The figure shows three views and two pictorial views of one solid part (mm, origin at its lowest corner). Answer the questions. Coordinates: 2 decimals unless noted, no trailing zeros. Write each loop counter-clockwise with the first axis right and the second up, starting at its lowest first coordinate (ties: lowest second). Pieces come first, ordered by that corner, then holes.
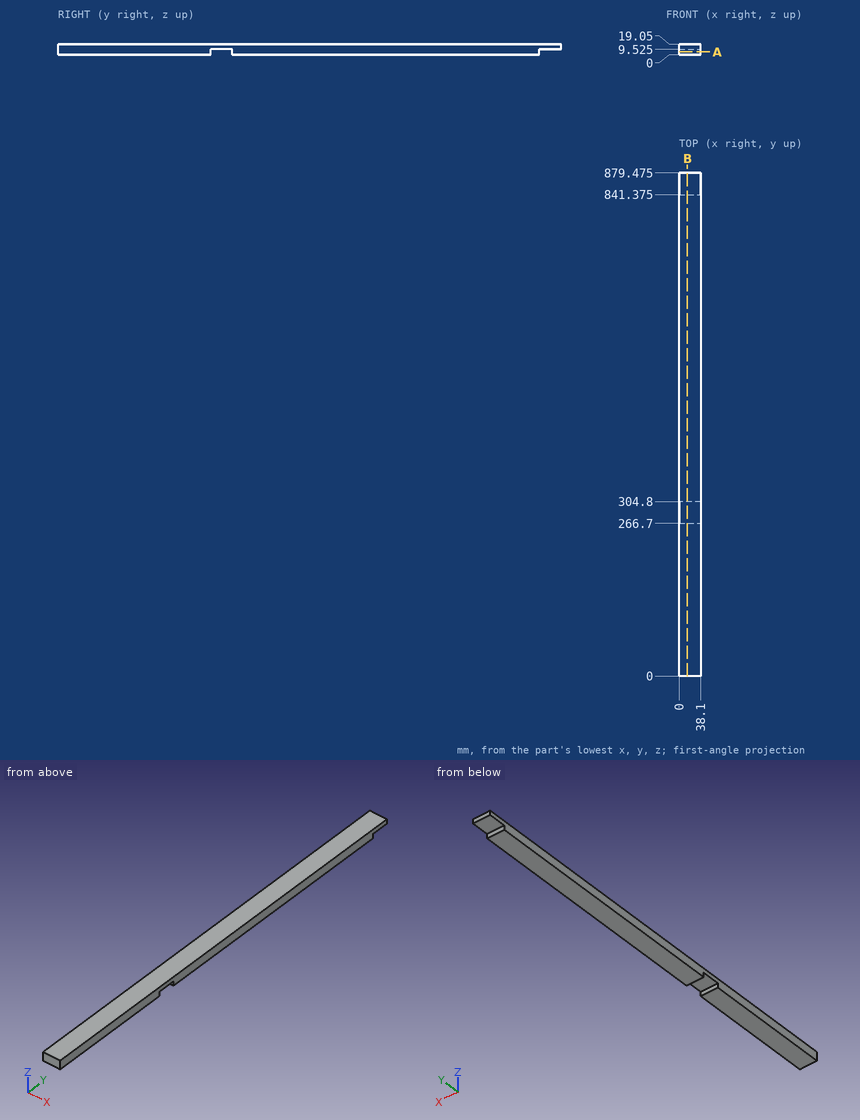
1. A flat-ended cylindrical pin translates along its axis: P1, Ø19, axis at x = 28, y = 295, coming from the -Z side (3 decimals). Find the tip coordinate at first contact, or state that the pin passes through.
Results found:
P1: stops at z = 9.525
2. Section A-A on z = 5.25 is taken. Give the vertices of the cut face in (x, y) (3 decimals).
Results found:
outline: (0, 0) - (38.1, 0) - (38.1, 266.7) - (0, 266.7) - close; (0, 304.8) - (38.1, 304.8) - (38.1, 841.375) - (0, 841.375) - close
3. Section B-B on x = 14.5 is taken. Give the vertices of the cut face in (y, z) (3 decimals), then the cut area to 3 significant figures.
Results found:
outline: (0, 0) - (266.7, 0) - (266.7, 9.525) - (304.8, 9.525) - (304.8, 0) - (841.375, 0) - (841.375, 9.525) - (879.475, 9.525) - (879.475, 19.05) - (0, 19.05) - close
area: 16,000 mm2
4. Find the intervals of material crossed by L1, parallel to Y at x = 22.5, z = 5.25 (3 decimals), in increasing order.
Results found:
L1: y = 0 to 266.7, 304.8 to 841.375
